```python
from build123d import *

# Parameters (mm, degrees)
F0_R     = 75.9892747742
F1_DEPTH = 25.4
F2_R     = 75.972189553
F3_DEPTH = 25.4
F4_R     = 76.4406104517
F5_DEPTH = 25.4
F7_D     = 12.7


with BuildPart() as f1:
    # F0 (on Front) → F1 (new body)
    with BuildSketch(Plane.XZ):
        Circle(F0_R)
    extrude(amount=F1_DEPTH)

    # F2 (on Right) → F3 (join)
    with BuildSketch(Plane.YZ):
        Circle(F2_R)
    extrude(amount=F3_DEPTH)

    # F4 (on Top) → F5 (join)
    with BuildSketch(Plane.XY):
        Circle(F4_R)
    extrude(amount=F5_DEPTH)

    # F7 (through all)
    with Locations(Plane(origin=(0, 0, 0), x_dir=(1, 0, 0), z_dir=(0, 1, 0))):
        with Locations((-20.7811314613, -58.2467317581)):
            Hole(F7_D / 2)


solid = f1.part
```
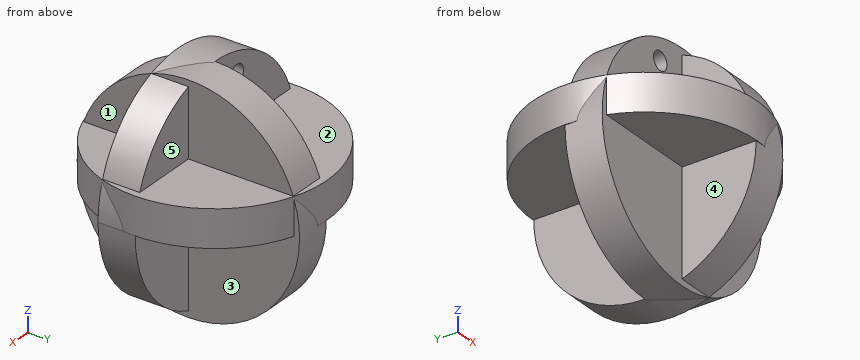
CAD build for the part. Positions are in the model's coordinates, mm. Face numbers are marked on the shaded views. A direction names the side the tool comes from. Coordinates: 2 decimals unless noted, no trailing zeros. Order: outer loops, then holes, each group sorted by start corner. A loop starts at its lowest first (then second) coordinate and runs counter-clockwise, first axis right, second up. Notation, with made-up numbers: M 43,39 L 52,39 A17 cw 52,71 Z; hole C -39.5,82.25 d1. An arc over 180 degrees is marked long. Answer as CSV lines item,"result".
1) 3-axis set-ups, long thin cutter, end or side, ignore diameter. For the marked faces 1, 2, 3, 4 and 5: which of +Z, -Z, +X, -X, +Y, -Y reach the whole face in a straight line?
Verdict:
face 1,"+Z, +X, -Y"
face 2,"+Z"
face 3,"-Z, +X, +Y"
face 4,"-Z, -X, -Y"
face 5,"+Z, +X, +Y"
2) Cut at D-D (z = -14). List the corners of the cut face in (x, y), then the cut area to 3 significant figures.
Verdict:
outline,"M -74.69,-25.4 L 0,-25.4 L 0,-74.67 L 25.4,-74.67 L 25.4,-25.4 L 74.69,-25.4 L 74.69,0 L 25.4,0 L 25.4,74.67 L 0,74.67 L 0,0 L -74.69,0 Z"
area,"6,940 mm2"
3) Flat gauge pins, fed straight in: P1, Ø6, axis at y = -42.5, z = 3.5, coming from the -X side; P2, Ø2, axis at y = -18, z = 20.5, coming from the +X side; P3, Ø10, axis at x = 56.5, y = -18.5, coming from the +Z side. Where does each tip first touch, or does it go through?
Verdict:
P1,"x = -65.44"
P2,"x = 74.53"
P3,"z = 55.88"
4) Drill centre lines: L1, parallel to Y at x = -42.5, z = -40; L2, parallel to X at y = 29, z = 30. Where is each one in solid material? Low to high. Write a range as from..to.
Verdict:
L1,"-25.4..0"
L2,"0..25.4"
5) Cut at B-B (y = -3). List the corners of the cut face in (x, z).
Verdict:
outline,"M -76.38,0 L -75.99,0 A75.99 ccw 3.41,-75.91 L 25.4,-75.91 L 25.4,-71.62 A75.99 ccw 75.99,0 L 76.38,0 L 76.38,25.4 L 71.62,25.4 A75.99 ccw 25.4,71.62 L 25.4,75.91 L 3.41,75.91 A75.99 ccw -71.62,25.4 L -76.38,25.4 Z; hole C -20.78,58.25 d12.7"
6) Cut at C-C (x = 17). List the corners of the cut face in (y, z), then the cut area to 3 significant figures.
Verdict:
outline,"M -74.53,14.75 A75.97 ccw -25.4,-71.6 L -25.4,-74.06 L -16.92,-74.06 A75.97 ccw 74.53,14.75 L 74.53,25.4 L 71.6,25.4 A75.97 ccw -16.92,74.06 L -25.4,74.06 L -25.4,71.6 A75.97 ccw -71.6,25.4 L -74.53,25.4 Z"
area,"18,200 mm2"
7) Cut at A-A (z = 55). List the corners of the cut face in (x, y).
Verdict:
outline,"M -52.43,-25.4 L -26.24,-25.4 L -26.24,0 L -52.43,0 Z; M -15.32,-25.4 L 0,-25.4 L 0,-52.41 L 25.4,-52.41 L 25.4,-25.4 L 52.43,-25.4 L 52.43,0 L 25.4,0 L 25.4,52.41 L 0,52.41 L 0,0 L -15.32,0 Z"
